Work out the finished part from the listing and answer in its coordinate system (mm). Give positions to 0.01 mm unless a question says otherwise; leave off trailing zeros. Loops run counter-clockwise (first coordinate to the right, second up) from the corner with the lowest first, then second, coordinate; pieces in that order, holes last. Notation, with made-up numbers: M 47.5,83.25 L 85.5,83.25 A24 cw 85.5,110.25 Z; hole C 16,56.5 d1. An arc over 180 degrees is marked long. Use a Markdown table: item, result.
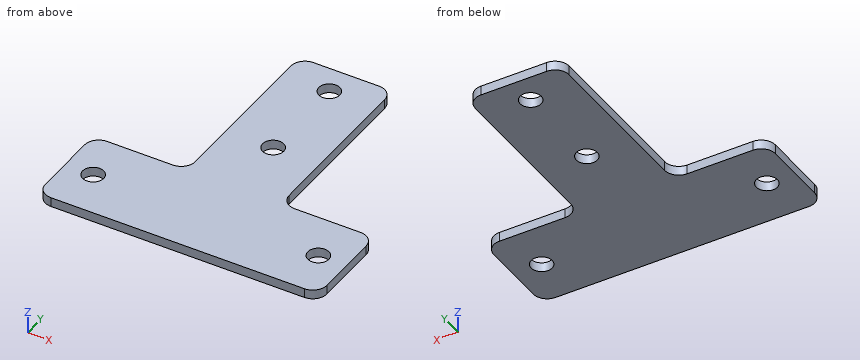
```python
from build123d import *

# Parameters (mm, degrees)
SKETCH_1_R             = 2.25
SM_BASE_FLANGE_1_DEPTH = 2


# Sheet-metal steps are written as plain solids
with BuildPart() as part:
    # Sketch 1 → 基体-法兰1 (new body)
    with BuildSketch(Plane.XY):
        with BuildLine():
            Line((-27, 0), (27, 0))
            ThreePointArc((27, 0), (29.121320344, 0.878679656), (30, 3))
            Line((30, 3), (30, 17))
            ThreePointArc((30, 17), (29.121320344, 19.121320344), (27, 20))
            Line((27, 20), (13, 20))
            ThreePointArc((13, 20), (10.878679656, 20.878679656), (10, 23))
            Line((10, 23), (10, 32.5))
            Line((10, 32.5), (10, 57))
            ThreePointArc((10, 57), (9.121320344, 59.121320344), (7, 60))
            Line((7, 60), (-7, 60))
            ThreePointArc((-7, 60), (-9.121320344, 59.121320344), (-10, 57))
            Line((-10, 57), (-10, 23))
            ThreePointArc((-10, 23), (-10.878679656, 20.878679656), (-13, 20))
            Line((-13, 20), (-27, 20))
            ThreePointArc((-27, 20), (-29.121320344, 19.121320344), (-30, 17))
            Line((-30, 17), (-30, 3))
            ThreePointArc((-30, 3), (-29.121320344, 0.878679656), (-27, 0))
        make_face()
        with Locations((-24, 10)):
            Circle(SKETCH_1_R, mode=Mode.SUBTRACT)
        with Locations(Location((24, 10, 0), (0, 0, 180))):
            Circle(SKETCH_1_R, mode=Mode.SUBTRACT)
        with Locations((0, 54)):
            Circle(SKETCH_1_R, mode=Mode.SUBTRACT)
        with Locations((0, 34)):
            Circle(SKETCH_1_R, mode=Mode.SUBTRACT)
    extrude(amount=-SM_BASE_FLANGE_1_DEPTH)


solid = part.part
```
(1) Given P1, Ø1, axis at x = 19.5, z = -1.5, coming from the +Y side; P2, Ø6, axis at x = 24, y = 10, coming from the -Z side; P3, Ø4, axis at x = 0, y = 54, coming from the +Z side, each flat-ended and moving along its own axis, determine where each tip first touches the part or whether it passes through.
Entries:
| item | result |
|---|---|
| P1 | stops at y = 20 |
| P2 | stops at z = -2 |
| P3 | passes through |
(2) A cutting plane is placed at B-B (y = 54). Write down the section's boundary in (x, z), and give its area (3 significant figures).
Entries:
| item | result |
|---|---|
| outline | M -10,-2 L -2.25,-2 L -2.25,0 L -10,0 Z; M 2.25,-2 L 10,-2 L 10,0 L 2.25,0 Z |
| area | 31.0 mm² |
(3) Consider probe 1 along Y at (x, z) = (0, -0.4); probe 2 along Y at (x, z) = (-1.5, -0.95); probe 3 along Y at (x, z) = (-24, -1.15). Determine where each line is inside the solid, lowest interval first. Write a range as [from, to].
Entries:
| item | result |
|---|---|
| probe 1 | y = [0, 31.75], [36.25, 51.75], [56.25, 60] |
| probe 2 | y = [0, 32.32], [35.68, 52.32], [55.68, 60] |
| probe 3 | y = [0, 7.75], [12.25, 20] |
(4) A cutting plane is placed at D-D (z = -0.7). Write down the section's boundary in (x, y), and give its area (3 significant figures).
Entries:
| item | result |
|---|---|
| outline | M -30,3 A3 ccw -27,0 L 27,0 A3 ccw 30,3 L 30,17 A3 ccw 27,20 L 13,20 A3 cw 10,23 L 10,57 A3 ccw 7,60 L -7,60 A3 ccw -10,57 L -10,23 A3 cw -13,20 L -27,20 A3 ccw -30,17 Z; hole C -24,10 d4.5; hole C 0,34 d4.5; hole C 0,54 d4.5; hole C 24,10 d4.5 |
| area | 1,930 mm² |
(5) A cutting plane is placed at A-A (x = 24). Write down the section's boundary in (y, z).
Entries:
| item | result |
|---|---|
| outline | M 0,-2 L 7.75,-2 L 7.75,0 L 0,0 Z; M 12.25,-2 L 20,-2 L 20,0 L 12.25,0 Z |
(6) A cutting plane is placed at C-C (y = 10). Write down the section's boundary in (x, z), and give its area (3 significant figures).
Entries:
| item | result |
|---|---|
| outline | M -30,-2 L -26.25,-2 L -26.25,0 L -30,0 Z; M -21.75,-2 L 21.75,-2 L 21.75,0 L -21.75,0 Z; M 26.25,-2 L 30,-2 L 30,0 L 26.25,0 Z |
| area | 102 mm² |
